Design review of the part built by this model. Coordinates are the model's own, in mm. Give positions to 0.01 mm unless a question says otherwise; leave off trailing zeros. Order: outer loops, then holes, each group sorted by start corner. A loop starts at its lowest first (then second) coordinate and runs counter-clockwise, first axis right, second up. Notation, with made-up numbers: M 76,6.25 L 101,6.25 A28 ccw 101,37.25 Z; hole C -3,74.25 d7. An arc over 180 degrees is marked long. Answer as a JSON object with one key per item and string values.
from build123d import *

# Parameters (mm, degrees)
CYLINDER006_R          = 3
CYLINDER006_DEPTH      = 10
CYLINDER006_ROLL_ANGLE = 90
ARRAY006_Z_COUNT       = 2
ARRAY006_Z_PITCH       = 20
CYLINDER005_R          = 2
CYLINDER005_DEPTH      = 6
CYLINDER005_ROLL_ANGLE = 90
ARRAY005_X_COUNT       = 2
ARRAY005_X_PITCH       = 26
ARRAY005_Z_COUNT       = 2
ARRAY005_Z_PITCH       = 26
BOX013_W               = 40
BOX013_H               = 60
BOX013_DEPTH           = 6
BOX013_ROLL_ANGLE      = 90


with BuildPart() as array006:
    # Cylinder006 → Cylinder006 (new body)
    with BuildSketch(Plane.XY):
        Circle(CYLINDER006_R)
    extrude(amount=CYLINDER006_DEPTH)


with BuildPart() as array006_1:
    # Cylinder006 roll: moved
    add(array006.part.rotate(Axis((0, 0, 0), (1, 0, 0)), CYLINDER006_ROLL_ANGLE))


with BuildPart() as array006_2:
    # Cylinder006 placement: moved
    add(array006_1.part.moved(Location((20, 0, 21))))

    # Array006 Z: Array006 ×2


with BuildPart() as array006_3:
    add(array006_2.part)
    with Locations(*[(0, 0, i * ARRAY006_Z_PITCH) for i in range(1, ARRAY006_Z_COUNT)]):
        add(array006_2.part)


with BuildPart() as array005:
    # Cylinder005 → Cylinder005 (new body)
    with BuildSketch(Plane.XY):
        Circle(CYLINDER005_R)
    extrude(amount=CYLINDER005_DEPTH)


with BuildPart() as array005_1:
    # Cylinder005 roll: moved
    add(array005.part.rotate(Axis((0, 0, 0), (1, 0, 0)), CYLINDER005_ROLL_ANGLE))


with BuildPart() as array005_2:
    # Cylinder005 placement: moved
    add(array005_1.part.moved(Location((7, 0, 19))))

    # Array005 X: Array005 ×2


with BuildPart() as array005_3:
    add(array005_2.part)
    with Locations(*[(i * ARRAY005_X_PITCH, 0, 0) for i in range(1, ARRAY005_X_COUNT)]):
        add(array005_2.part)

    # Array005 Z: Array005 ×2


with BuildPart() as array005_4:
    add(array005_3.part)
    with Locations(*[(0, 0, i * ARRAY005_Z_PITCH) for i in range(1, ARRAY005_Z_COUNT)]):
        add(array005_3.part)


with BuildPart() as obj1:
    # Box013 → Box013 (new body)
    with BuildSketch(Plane.XY):
        with Locations((20, 30)):
            Rectangle(BOX013_W, BOX013_H)
    extrude(amount=BOX013_DEPTH)


with BuildPart() as obj1_1:
    # Box013 roll: moved
    add(obj1.part.rotate(Axis((0, 0, 0), (1, 0, 0)), BOX013_ROLL_ANGLE))


with BuildPart() as obj1_2:
    # Box013 placement: moved
    add(obj1_1.part)

    # Cut006: cut Array005
    add(array005_4.part, mode=Mode.SUBTRACT)

    # Cut007: cut Array006
    add(array006_3.part, mode=Mode.SUBTRACT)


with BuildPart() as obj1_3:
    # Cut007 placement: moved
    add(obj1_2.part.moved(Location((2, -120, -19))))


solid = obj1_3.part
(1) To check wall thickness, follow L1, parallel to Z at x = 9, y = -121.15; L2, parallel to Z at x = 22, y = -123.15; L3, parallel to X at y = -123.4, z = 22. State the ranges of each line that lie inside material, in increasing order. Write a range as from..to.
Checked values:
{"L1": "z = -19..-2, 2..24, 28..41", "L2": "z = -19..-1, 5..19, 25..41", "L3": "x = 2..19, 25..42"}
(2) Draft analysis for pull direction Z (two halves, no side actions). For faces 1 (the cylindrical face through (19, -123, 2)), 2 (the flat face through (22, -123, -19)), 3 (the flat face through (42, -123, 11)), state which applies: +Z half, -Z half, draft (parallel to the pull), parting line (faces both ways), or undercut.
Checked values:
{"face 1": "undercut", "face 2": "-Z half", "face 3": "draft"}
(3) We need section D-D (z = 0). Write out the cut boundary in (x, y).
Checked values:
{"outline": "M 2,-126 L 7,-126 L 7,-120 L 2,-120 Z; M 11,-126 L 19.76,-126 L 19.76,-120 L 11,-120 Z; M 24.24,-126 L 33,-126 L 33,-120 L 24.24,-120 Z; M 37,-126 L 42,-126 L 42,-120 L 37,-120 Z"}
(4) We need section B-B (x = 22). Write out the cut boundary in (y, z), plus the area to 3 significant figures.
Checked values:
{"outline": "M -126,-19 L -120,-19 L -120,-1 L -126,-1 Z; M -126,5 L -120,5 L -120,19 L -126,19 Z; M -126,25 L -120,25 L -120,41 L -126,41 Z", "area": "288 mm^2"}
(5) We need section C-C (y = -124.1). Write out the cut boundary in (x, z), plus the area to 3 significant figures.
Checked values:
{"outline": "M 2,-19 L 42,-19 L 42,41 L 2,41 Z; hole C 9,0 d4; hole C 9,26 d4; hole C 22,2 d6; hole C 22,22 d6; hole C 35,0 d4; hole C 35,26 d4", "area": "2,290 mm^2"}
(6) We need section A-A (z = 26). Write out the cut boundary in (x, y), plus the area to 3 significant figures.
Checked values:
{"outline": "M 2,-126 L 7,-126 L 7,-120 L 2,-120 Z; M 11,-126 L 33,-126 L 33,-120 L 11,-120 Z; M 37,-126 L 42,-126 L 42,-120 L 37,-120 Z", "area": "192 mm^2"}
